Verification items for the finished model (mm, model axes). Face numbers are marked on the shaded views. Coordinates: 2 decimals unless noted, no trailing zeros. Write each loop counter-clockwise with the first axis right and the second up, starting at its lowest first coordinate (ties: lowest second). Pieces come first, ordered by that corner, then holes. Notation, with made-up numbers: (-23.75, 20.25) -> (34.25, 20.25) arc R15 cw to (34.25, 31.25) -> close; hole circle Ø5 at (-36, 12.5). An arc over 180 degrees is marked (long way). Use a Markdown table: item, result. Add a question column.
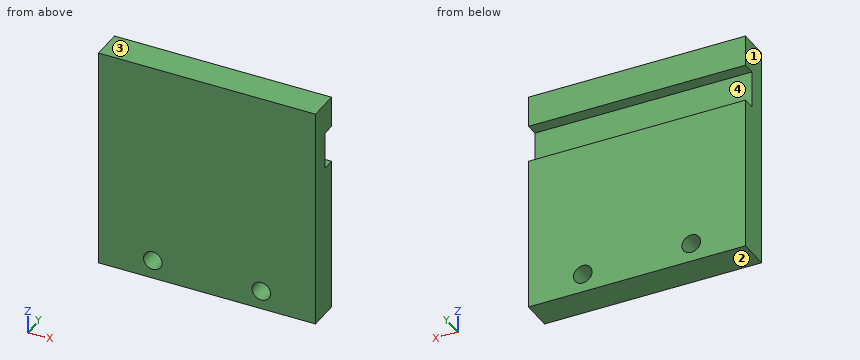
Autodesk Inventor part; units mm, degrees
ref_plane "YZ Plane" through (0, 0, 0) normal (1, 0, 0) x (0, 1, 0)
ref_plane "XZ Plane" through (0, 0, 0) normal (0, 1, 0) x (-1, 0, 0)
ref_plane "XY Plane" through (0, 0, 0) normal (0, 0, 1) x (1, 0, 0)
sketch "Sketch1" plane through (0, 0, 0) normal (0, 1, 0) x (-1, 0, 0)
  line L0 (0, 0) -> (35, 0)
  line L1 (35, 0) -> (35, 6)
  line L2 (0, 6) -> (35, 6)
  line L3 (0, 0) -> (0, 6)
  line L4 (0, 6) -> (0, 0)
  line L5 (0, 3) -> (35, 3)
  line L6 (17.5, 3) -> (35, 3)
  line L7 (17.5, 3) -> (0, 3)
  point P0 (17.5, 0)
  point P1 (8.75, 3)
  point P2 (26.25, 3)
extrude "Extrusion1" add sketch "Sketch1" along normal blind 5
sketch "Sketch2" plane through (-35, 0, 6) normal (0, 0, 1) x (1, 0, 0)
  line L0 (0, 0) -> (35, 0)
  line L1 (35, 0) -> (35, 5)
  line L2 (0, 5) -> (35, 5)
  line L3 (0, 0) -> (0, 5)
extrude "Extrusion2" add sketch "Sketch2" along normal blind 30
sketch "Sketch3" plane through (0, 5, 0) normal (0, 1, 0) x (1, 0, 0)
  line L0 (0, 0) -> (0, -36)
  line L1 (0, 0) -> (-35, 0)
  line L2 (-35, 0) -> (-35, -36)
  line L3 (0, -36) -> (-35, -36)
  line L4 (-35, 0) -> (-35, -36)
  line L5 (-35, -31) -> (0, -31)
  line L6 (0, -31) -> (0, -25)
  line L7 (0, -25) -> (-35, -25)
  line L8 (-35, -25) -> (-35, -31)
  dimension "d4" = 5
  dimension "d5" = 25
extrude "Extrusion3" cut sketch "Sketch3" against normal blind 2 contours L0 L5 L2 L7
sketch "Sketch4" plane through (0, 0, 0) normal (0, -1, 0) x (1, 0, 0)
  line L0 (-35, 0) -> (0, 0)
  line L1 (0, 0) -> (0, 6)
  line L2 (-35, 6) -> (0, 6)
  line L3 (-35, 0) -> (-35, 6)
  line L4 (-35, 6) -> (-35, 0)
  line L5 (-35, 3) -> (0, 3)
  line L6 (-17.5, 3) -> (0, 3)
  line L7 (-17.5, 3) -> (-35, 3)
  point P0 (0, 0)
  point P1 (-17.5, 0)
  point P2 (-8.75, 3)
  point P3 (-26.25, 3)
hole "Hole1" at (-8.75, 0, 3) at (-26.25, 0, 3) direction (0, 1, 0) diameter 3 depth 8 tip angle 118
properties part number "angle_clip" material "ABS Plastic"
1) Cross-section at A-A on z = 3. Record the boundary of the cut face in (x, y), then the cut area to 3 significant figures.
2) Gauge pin test, flat ends, axial feed: pin 1 (6.5 mm diameter, centred on x = -14.5, z = 27.5, fed in from +Y); pin 2 (2.5 mm diameter, centred on x = -8.75, z = 3, fed in from -Y). Record the tip position at first contact, or that the pin passes through.
3) Thickness scan on L1, parallel to X at y = 3.7, z = 3; L2, parallel to Z at x = -8.75, y = 1.4; L3, parallel to Z at x = -8.75, y = 3.6. Record the ranges inside material, lowest first.
4) Release check for a two-part mould opening along Z. For the marked faces 1, 2, 3 and 4 record: released by +Z, released by -Z, zero draft, split by the parting line, or undercut.
5) Cross-section at B-B on x = -26.25. Record the boundary of the cut face in (y, z), then the cut area to 3 significant figures.
Returned:
| question | item | result |
|---|---|---|
| 1 | outline | (-35, 0) -> (-27.75, 0) -> (-27.75, 5) -> (-35, 5) -> close; (-24.75, 0) -> (-10.25, 0) -> (-10.25, 5) -> (-24.75, 5) -> close; (-7.25, 0) -> (0, 0) -> (0, 5) -> (-7.25, 5) -> close |
| 1 | area | 145 mm² |
| 2 | pin 1 | stops at y = 5 |
| 2 | pin 2 | passes through |
| 3 | L1 | x = -35 to -27.75, -24.75 to -10.25, -7.25 to 0 |
| 3 | L2 | z = 0 to 1.5, 4.5 to 36 |
| 3 | L3 | z = 0 to 1.5, 4.5 to 25, 31 to 36 |
| 4 | face 1 | zero draft |
| 4 | face 2 | released by -Z |
| 4 | face 3 | released by +Z |
| 4 | face 4 | undercut |
| 5 | outline | (0, 0) -> (5, 0) -> (5, 1.5) -> (0, 1.5) -> close; (0, 4.5) -> (5, 4.5) -> (5, 25) -> (3, 25) -> (3, 31) -> (5, 31) -> (5, 36) -> (0, 36) -> close |
| 5 | area | 153 mm² |
